```python
from build123d import *

# Parameters (mm, degrees)
F0_R     = 49.9999
F1_DEPTH = 79.99984
F2_R     = 3.175
F3_DEPTH = 120.99898
F4_DEPTH = 120.99898
F5_R     = 5.48005
F6_DEPTH = 4.064
F7_R     = 5.4864
F8_DEPTH = 4.064


with BuildPart() as f1:
    # F0 (on Front) → F1 (new body)
    with BuildSketch(Plane.XZ):
        with BuildLine():
            Line((-85.99932, -68.295799), (0, -68.295799))
            Line((0, -68.295799), (85.99932, -68.295799))
            Line((85.99932, -68.295799), (85.99932, -51.370141))
            Line((85.99932, -51.370141), (64.99987, -51.370141))
            Line((64.99987, -51.370141), (64.99987, 23.628439))
            Line((64.99987, 23.628439), (54.628692, 23.628439))
            ThreePointArc((54.628692, 23.628439), (0, 52.702181), (-54.628692, 23.628439))
            Line((-54.628692, 23.628439), (-64.99987, 23.628439))
            Line((-64.99987, 23.628439), (-64.99987, -51.370141))
            Line((-64.99987, -51.370141), (-85.99932, -51.370141))
            Line((-85.99932, -51.370141), (-85.99932, -68.295799))
        make_face()
        with Locations((0.550864, -7.294665)):
            Circle(F0_R, mode=Mode.SUBTRACT)
    extrude(amount=F1_DEPTH)

    # F2 (on face) → F3 (cut, through all)
    with BuildSketch(Plane(origin=(0, 0, -68.295799), x_dir=(1, 0, 0), z_dir=(0, 0, -1))):
        with Locations((-75.49896, 66.29781)):
            Circle(F2_R)
        with Locations((-75.49896, 39.99992)):
            Circle(F2_R)
        with Locations((-75.49896, 13.70203)):
            Circle(F2_R)
        with Locations((75.49896, 66.29781)):
            Circle(F2_R)
        with Locations((75.49896, 39.99992)):
            Circle(F2_R)
        with Locations((75.49896, 13.70203)):
            Circle(F2_R)
    extrude(amount=-F3_DEPTH, mode=Mode.SUBTRACT)

    # F2 (on face) → F4 (cut, through all)
    with BuildSketch(Plane(origin=(0, 0, -68.295799), x_dir=(1, 0, 0), z_dir=(0, 0, -1))):
        with Locations((-75.49896, 66.29781)):
            Circle(F2_R)
        with Locations((-75.49896, 39.99992)):
            Circle(F2_R)
        with Locations((-75.49896, 13.70203)):
            Circle(F2_R)
        with Locations((75.49896, 66.29781)):
            Circle(F2_R)
        with Locations((75.49896, 39.99992)):
            Circle(F2_R)
        with Locations((75.49896, 13.70203)):
            Circle(F2_R)
    extrude(amount=-F4_DEPTH, mode=Mode.SUBTRACT)

    # F5 (on face) → F6 (cut)
    with BuildSketch(Plane.XY.offset(-51.370141)):
        with Locations((75.49896, -13.70203)):
            Circle(F5_R)
        with Locations((75.49896, -39.99992)):
            Circle(F5_R)
        with Locations((75.49896, -66.29781)):
            Circle(F5_R)
    extrude(amount=-F6_DEPTH, mode=Mode.SUBTRACT)

    # F7 (on face) → F8 (cut)
    with BuildSketch(Plane.XY.offset(-51.370141)):
        with Locations((-75.49896, -13.70203)):
            Circle(F7_R)
        with Locations((-75.49896, -39.99992)):
            Circle(F7_R)
        with Locations((-75.49896, -66.29781)):
            Circle(F7_R)
    extrude(amount=-F8_DEPTH, mode=Mode.SUBTRACT)


solid = f1.part
```
Input: part model. Units: mm. Frame: model coordinates. A direction names the side the tool comes from. Give positions to 0.01 mm unless a question says otherwise; leave off trailing zeros. Order: outer loops, then holes, each group sorted by start corner. A loop starts at its lowest first (then second) coordinate and runs counter-clockwise, first axis right, second up. Notation, with made-up numbers: M 79,37 L 89,37 A19 ccw 89,59 Z; hole C 4.25,27.5 d11. An arc over 180 degrees is marked long. Return JSON: item names as keys, results as strings.
Item 1: Pull-direction query (X, two-part tool) for faces 6 (the cylindrical face through (72.98, -11.77, -61.96)), 7 (the flat face through (-1, -39, -68.296)), 8 (the flat face through (-65, -39, -13)); classes: +X half, -X half, draft (parallel to the pull), parting line (faces both ways), or undercut.
Solutions:
{"face 6": "undercut", "face 7": "draft", "face 8": "-X half"}
Item 2: Cut plane B-B (z = 32.5). Return loops of the section in (x, y).
Solutions:
{"outline": "M -47.46,-80 L -29.72,-80 L -29.72,0 L -47.46,0 Z; M 30.82,-80 L 47.46,-80 L 47.46,0 L 30.82,0 Z"}
Item 3: Cut plane A-A (x = 16.5). Return loops of the section in (y, z).
Solutions:
{"outline": "M -80,-68.3 L 0,-68.3 L 0,-54.68 L -80,-54.68 Z; M -80,40.09 L 0,40.09 L 0,50.6 L -80,50.6 Z"}
Item 4: Ray query, probe 1 along X at (y, z) = (-75, -5.5); probe 2 along Z at (x, y) = (-63, -9.5); probe 3 along Z at (x, y) = (39.5, -46). Return the intervals inside material, ascending.
Solutions:
{"probe 1": "-65 to -49.42, 50.52 to 65", "probe 2": "-68.3 to 23.63", "probe 3": "-68.3 to -38.65, 24.06 to 39.54"}
Item 5: Cut plane D-D (z = 45). Return loops of the section in (x, y).
Solutions:
{"outline": "M -30.91,-80 L 30.91,-80 L 30.91,0 L -30.91,0 Z"}
Item 6: Cut plane C-C (y = -47.5). Return loops of the section in (x, z).
Solutions:
{"outline": "M -86,-68.3 L 86,-68.3 L 86,-51.37 L 65,-51.37 L 65,23.63 L 54.63,23.63 A65.86 ccw -54.63,23.63 L -65,23.63 L -65,-51.37 L -86,-51.37 Z; hole C 0.55,-7.29 d100"}
Item 7: Access query for faces 1 (the flat face through (-82, -39, -51.37)), 2 (the flat face through (83, -39, -51.37)), 3 (the flat face through (-73.1, -42.4, -55.434)), 4 (the cylindrical face through (75.086, -69.446, -61.955)), 5 (the flat face through (-85.999, -39, -60)). Directions: +Z, -Z, +X, -X, +Y, -Y. A direction counts if a zero-diameter tool reaches every point of the face in a straight line with its end or side. Return the directions, or none.
Solutions:
{"face 1": "+Z, -X, +Y, -Y", "face 2": "+Z, +X, +Y, -Y", "face 3": "+Z", "face 4": "+Z, -Z", "face 5": "+Z, -Z, -X, +Y, -Y"}
Item 8: First-contact query: P1, Ø12, axis at x = 73, y = -67, coming from the +Z side; P2, Ø11.5, axis at x = -58, y = -55.5, coming from the +Z side; P3, Ø3.5, axis at x = -78, y = -41.5, coming from the +Z side. Flat tips, straight axial feed; report the tip coordinate or a pass-through.
Solutions:
{"P1": "z = -51.37", "P2": "z = 26.94", "P3": "z = -55.43"}
